Study the drawing (mm; zero at the part's minimum x, y, z) and answer. A direction names the side the tool comes from. Round coordinates to 2 decimals unless told otherwise and drop trailing zeros. Loops run counter-clockwise (first coordinate to the right, second up) from the corner with the lowest first, then second, coordinate; pieces in that order, holes last. Notation, with made-up numbers: M 18,13 L 56,13 A12 ccw 56,32 Z; hole C 58.25,-0.75 d8. An arc over 180 degrees is marked long. Write each question's results on one line, items separated by ' | '.
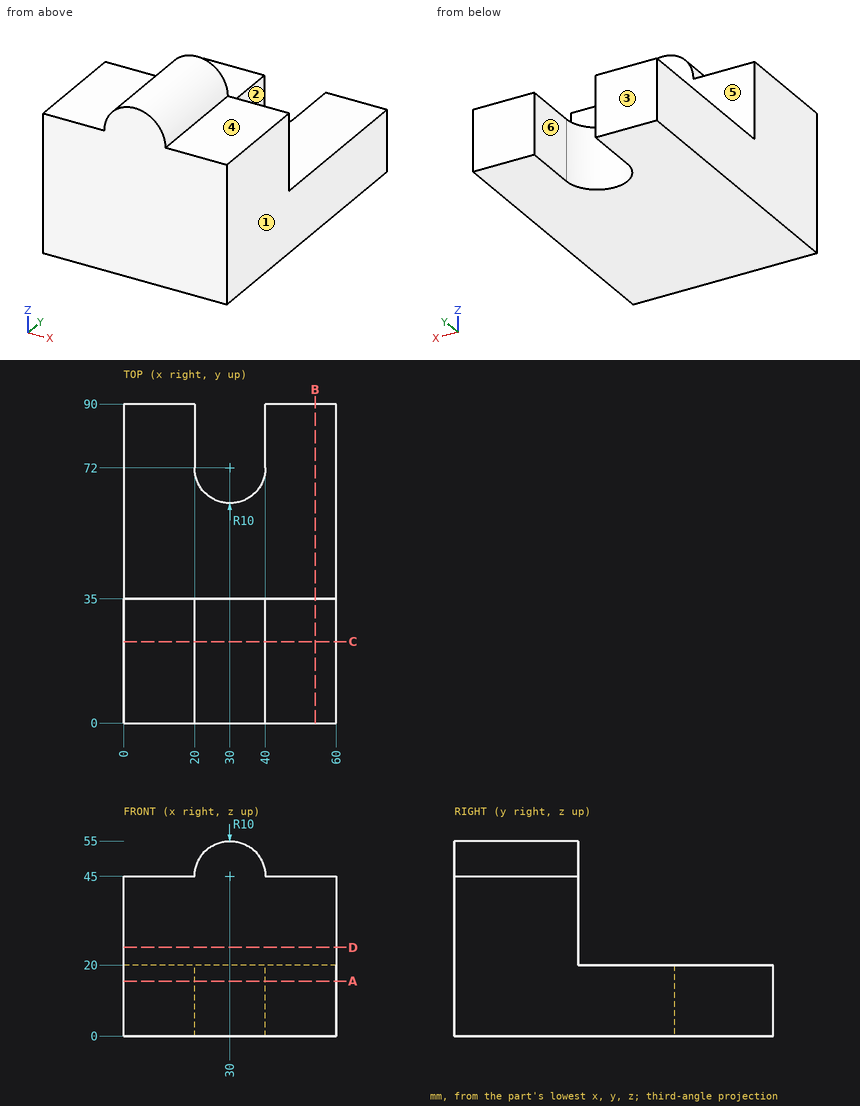
Item 1: The part is cut by section B-B (x = 54). Determine the outline of the cut face in (y, z), plus the area to 4 significant figures.
Outcome:
outline: M 0,0 L 90,0 L 90,20 L 35,20 L 35,45 L 0,45 Z | area: 2,675 mm2
Item 2: Straight lines are drawn through the part: line 1 (X direction, y = 73.5, z = 7); line 2 (Z direction, x = 10, y = 51); line 3 (Z direction, x = 30.5, y = 8.5). For each, find the intervals that lie inside material, in ascending order.
Outcome:
line 1: x = 0 to 20, 40 to 60 | line 2: z = 0 to 20 | line 3: z = 0 to 54.99
Item 3: For the marked faces 4, 5 and 6, determine the directions among +Z, -Z, +X, -X, +Y, -Y from which every point of the face is accessible in a straight line to the end or side of a thin tool.
Outcome:
face 4: +Z, +X, +Y, -Y | face 5: +Z, +X, -X, +Y | face 6: +Z, -Z, +Y
Item 4: The part is cut by section D-D (z = 25). Determine the outline of the cut face in (x, y).
Outcome:
outline: M 0,0 L 60,0 L 60,35 L 0,35 Z
Item 5: Flat-ended cylindrical pins translate along their axes: pin 1 (22 mm diameter, centred on x = 53, y = 25, fed in from +Z); pin 2 (8 mm diameter, centred on x = 18, y = 44, fed in from +Z); pin 3 (4 mm diameter, centred on x = 15, z = 48.5, fed in from +Y); pin 4 (22 mm diameter, centred on x = 13.5, y = 9.5, fed in from +Z). Find the tip coordinate at first contact, or state that the pin passes through.
Outcome:
pin 1: stops at z = 45 | pin 2: stops at z = 20 | pin 3: passes through | pin 4: stops at z = 53.35
Item 6: The part is cut by section A-A (z = 15.5). Determine the outline of the cut face in (x, y).
Outcome:
outline: M 0,0 L 60,0 L 60,90 L 40,90 L 40,72 A10 cw 20,72 L 20,90 L 0,90 Z
Item 7: The part is cut by section C-C (y = 23). Determine the outline of the cut face in (x, z).
Outcome:
outline: M 0,0 L 60,0 L 60,45 L 40,45 A10 ccw 20,45 L 0,45 Z
Item 8: The mould has two halves that part along X. Classify the marked faces 1, 2 and 3: pulls with the +X half, pulls with the -X half, needs draft (parallel to the pull), parting line crosses it, or undercut.
Outcome:
face 1: pulls with the +X half | face 2: undercut | face 3: needs draft
